from build123d import *

# Parameters (mm, degrees)
SKETCH_1_W                = 86
SKETCH_1_H                = 63
EXTRUDE_1_DEPTH           = 2
SKETCH_2_W                = 86
SKETCH_2_H                = 63
SKETCH_2_W_2              = 82
SKETCH_2_H_2              = 59
EXTRUDE_3_DEPTH           = 52.6
SKETCH_4_W                = 82
SKETCH_4_H                = 17.6
CUT_EXTRUDE_1_DEPTH       = 52.6
SKETCH_5_R                = 1.6
SKETCH_5_R_2              = 4.6
CUT_EXTRUDE_2_DEPTH       = 2
SKETCH_7_R                = 1.6
CUT_EXTRUDE_6_DEPTH       = 2
SKETCH_8_R                = 1.6
SKETCH_8_R_2              = 1.516132991
CUT_EXTRUDE_7_DEPTH       = 2
SKETCH_9_W                = 63
SKETCH_9_H                = 54.6
EXTRUDE_4_DEPTH           = 5
SKETCH_10_R               = 1.6
SKETCH_10_R_2             = 4.6
CUT_EXTRUDE_8_DEPTH       = 5
CUT_EXTRUDE_START         = -5
SKETCH_11_R               = 1.6
SKETCH_11_R_2             = 4.6
CUT_EXTRUDE_9_DEPTH       = 5
SKETCH_12_W               = 5
SKETCH_12_H               = 15.6
EXTRUDE_5_DEPTH           = 2
SKETCH_13_R               = 2.787491564
CUT_EXTRUDE_10_DEPTH      = 2
SKETCH_14_R               = 3
CUT_EXTRUDE_11_DEPTH      = 2
SKETCH_16_W               = 9
SKETCH_16_H               = 3.75891244
SKETCH_16_H_2             = 3.76
EXTRUDE_6_DEPTH           = 6
CUT_EXTRUDE_15_DEPTH      = 80.341453127
CUT_EXTRUDE_15_DEPTH_BACK = 80.341453127
SKETCH_17_R               = 1.6
SKETCH_18_W               = 9
SKETCH_18_H               = 6
SKETCH_18_R               = 1.6
EXTRUDE_7_DEPTH           = 3.76


with BuildPart() as part:
    # 草图1 → 凸台-拉伸1 (new body)
    with BuildSketch(Plane(origin=(0, 0, 0), x_dir=(1, 0, 0), z_dir=(0, 1, 0))):
        Rectangle(SKETCH_1_W, SKETCH_1_H)
    extrude(amount=EXTRUDE_1_DEPTH)

    # 草图2 → 凸台-拉伸3 (add)
    with BuildSketch(Plane(origin=(0, 2, 0), x_dir=(1, 0, 0), z_dir=(0, 1, 0))):
        Rectangle(SKETCH_2_W, SKETCH_2_H)
        Rectangle(SKETCH_2_W_2, SKETCH_2_H_2, mode=Mode.SUBTRACT)
    extrude(amount=EXTRUDE_3_DEPTH)

    # 草图4 → 切除-拉伸1 (cut)
    with BuildSketch(Plane.XY.offset(-29.5)):
        with Locations((0, 45.8)):
            Rectangle(SKETCH_4_W, SKETCH_4_H)
    extrude(amount=-CUT_EXTRUDE_1_DEPTH, mode=Mode.SUBTRACT)

    # 草图5 → 切除-拉伸2 (cut)
    with BuildSketch(Plane(origin=(43, 0, 0), x_dir=(0, 0, -1), z_dir=(1, 0, 0))):
        with Locations((-17.5, 16.95452537)):
            Circle(SKETCH_5_R)
        with Locations((17.5, 16.95452537)):
            Circle(SKETCH_5_R)
        with Locations((0, 8.95452537)):
            Circle(SKETCH_5_R_2)
    extrude(amount=-CUT_EXTRUDE_2_DEPTH, mode=Mode.SUBTRACT)

    # 草图7 → 切除-拉伸6 (cut)
    with BuildSketch(Plane(origin=(0, 2, 0), x_dir=(1, 0, 0), z_dir=(0, 1, 0))):
        with Locations(Location((-38.17, 6.16, 0), (0, 0, 270))):
            Circle(SKETCH_7_R)
        with Locations(Location((-38.17, -26.73, 0), (0, 0, 270))):
            Circle(SKETCH_7_R)
        with Locations(Location((36.38, -26.73, 0), (0, 0, 270))):
            Circle(SKETCH_7_R)
    extrude(amount=-CUT_EXTRUDE_6_DEPTH, mode=Mode.SUBTRACT)

    # 草图8 → 切除-拉伸7 (cut)
    with BuildSketch(Plane(origin=(0, 2, 0), x_dir=(1, 0, 0), z_dir=(0, 1, 0))):
        with Locations(Location((-39, 1.715, 0), (0, 0, 270))):
            Circle(SKETCH_8_R)
        with Locations(Location((21, -22.285, 0), (0, 0, 270))):
            Circle(SKETCH_8_R)
        with Locations(Location((-39, -22.285, 0), (0, 0, 270))):
            Circle(SKETCH_8_R_2)
        with Locations(Location((21, 1.715, 0), (0, 0, 270))):
            Circle(SKETCH_8_R)
    extrude(amount=-CUT_EXTRUDE_7_DEPTH, mode=Mode.SUBTRACT)

    # 草图9 → 凸台-拉伸4 (add)
    with BuildSketch(Plane(origin=(43, 0, 0), x_dir=(0, 0, -1), z_dir=(1, 0, 0))):
        with Locations((0, 27.3)):
            Rectangle(SKETCH_9_W, SKETCH_9_H)
    extrude(amount=EXTRUDE_4_DEPTH)

    # 草图10 → 切除-拉伸8 (cut)
    with BuildSketch(Plane(origin=(48, 0, 0), x_dir=(0, 0, -1), z_dir=(1, 0, 0))):
        with Locations((-17.5, 16.95452537)):
            Circle(SKETCH_10_R)
        with Locations((0, 8.95452537)):
            Circle(SKETCH_10_R_2)
        with Locations((17.5, 16.95452537)):
            Circle(SKETCH_10_R)
    extrude(amount=-CUT_EXTRUDE_8_DEPTH, mode=Mode.SUBTRACT)

    # 草图11 → 切除-拉伸9 (cut)
    with BuildSketch(Plane.ZY.offset(-41).offset(CUT_EXTRUDE_START)):
        Polygon((29.5, 52.6), (-31.5, 52.6), (-31.5, 37), (-29.5, 37), (-29.5, 2), (29.5, 2), align=None)
        with Locations(Location((-17.5, 16.95452537, 0), (0, 0, 180))):
            Circle(SKETCH_11_R, mode=Mode.SUBTRACT)
        with Locations(Location((0, 8.95452537, 0), (0, 0, 180))):
            Circle(SKETCH_11_R_2, mode=Mode.SUBTRACT)
        with Locations(Location((17.5, 16.95452537, 0), (0, 0, 180))):
            Circle(SKETCH_11_R, mode=Mode.SUBTRACT)
    extrude(amount=CUT_EXTRUDE_9_DEPTH, mode=Mode.SUBTRACT)

    # 草图12 → 凸台-拉伸5 (add)
    with BuildSketch(Plane(origin=(0, 0, -31.5), x_dir=(-1, 0, 0), z_dir=(0, 0, -1))):
        with Locations((-43.5, 44.8)):
            Rectangle(SKETCH_12_W, SKETCH_12_H)
    extrude(amount=-EXTRUDE_5_DEPTH)

    # 草图13 → 切除-拉伸10 (cut)
    with BuildSketch(Plane(origin=(48, 0, 0), x_dir=(0, 0, -1), z_dir=(1, 0, 0))):
        with Locations((24.963130904, 7.208902204)):
            Circle(SKETCH_13_R)
    extrude(amount=-CUT_EXTRUDE_10_DEPTH, mode=Mode.SUBTRACT)

    # 草图14 → 切除-拉伸11 (cut)
    with BuildSketch(Plane(origin=(0, 0, -31.5), x_dir=(-1, 0, 0), z_dir=(0, 0, -1))):
        with Locations((-28.059363277, 7.365425106)):
            Circle(SKETCH_14_R)
    extrude(amount=-CUT_EXTRUDE_11_DEPTH, mode=Mode.SUBTRACT)

    # 草图16 → 凸台-拉伸6 (add)
    with BuildSketch(Plane(origin=(0, 0, -31.5), x_dir=(-1, 0, 0), z_dir=(0, 0, -1))):
        with Locations((34.110668407, 1.87945622)):
            Rectangle(SKETCH_16_W, SKETCH_16_H)
        with Locations((-7.158197826, 1.88)):
            Rectangle(SKETCH_16_W, SKETCH_16_H_2)
    extrude(amount=EXTRUDE_6_DEPTH)

    # 草图17 → 切除-拉伸15 (cut, two sides: drawn at the far end of the back side and taken through both)
    with BuildSketch(Plane(origin=(0, 3.75891244, 0), x_dir=(1, 0, 0), z_dir=(0, 1, 0)).offset(-CUT_EXTRUDE_15_DEPTH_BACK)):
        with Locations(Location((-34.110668407, 34.625200871, 0), (0, 0, 180))):
            Circle(SKETCH_17_R)
        with Locations(Location((7.158197826, 34.625200871, 0), (0, 0, 180))):
            Circle(SKETCH_17_R)
    extrude(amount=CUT_EXTRUDE_15_DEPTH + CUT_EXTRUDE_15_DEPTH_BACK, mode=Mode.SUBTRACT)

    # 草图18 → 凸台-拉伸7 (add)
    # profile 1 of 2: a face of its own
    with BuildSketch(Plane.XZ):
        with Locations((7.158197826, 34.5)):
            Rectangle(SKETCH_18_W, SKETCH_18_H)
        with Locations(Location((7.158197826, 34.625200871, 0), (0, 0, 270))):
            Circle(SKETCH_18_R, mode=Mode.SUBTRACT)
    # profile 2 of 2: a face of its own
    with BuildSketch(Plane.XZ):
        with Locations((-34.110668407, 34.5)):
            Rectangle(SKETCH_18_W, SKETCH_18_H)
        with Locations(Location((-34.110668407, 34.625200871, 0), (0, 0, 270))):
            Circle(SKETCH_18_R, mode=Mode.SUBTRACT)
    extrude(amount=-EXTRUDE_7_DEPTH)


solid = part.part
Can you work these out from the model? Positions are in its coordinate system, mm. A direction names the side the tool comes from. Give positions to 0.01 mm unless a question says otherwise; leave off trailing zeros. Loops run counter-clockwise (first coordinate to the right, second up) from the corner with the lowest first, then second, coordinate; pieces in that order, holes last. Notation, with made-up numbers: (-18, -4.5) - (12, -4.5) arc R15 cw to (12, 15.5) - close; hole circle Ø2 at (22.25, 30). An arc over 180 degrees is marked (long way). Answer as a JSON object with one key per item and string values.
Q1. If we mould it in two halves opening along Z, with no side actions, what happens to faces 1 (the cylindrical face through (-40.48, 1.01, 21.96)), 2 (the cylindrical face through (-36.584, 1.014, -6.368)), 3 (the flat face through (41, 53, -8)), 4 (the flat face through (-34, 2, -37.5))? For each: pulls with the +Z half, pulls with the -Z half, needs draft (parallel to the pull), parting line crosses it, or undercut.
Geometry says:
{"face 1": "undercut", "face 2": "undercut", "face 3": "needs draft", "face 4": "pulls with the -Z half"}
Q2. Imagine slicing it at A-A on z = 17.5. Write out the boundary of the cut face in (x, y), plus the area to 3 significant figures.
Geometry says:
{"outline": "(-43, 0) - (48, 0) - (48, 15.35) - (46, 15.35) - (46, 2) - (-41, 2) - (-41, 54.6) - (-43, 54.6) - close; (41, 52.6) - (46, 52.6) - (46, 18.55) - (48, 18.55) - (48, 54.6) - (41, 54.6) - close", "area": "396 mm²"}
Q3. If I drill on L1, parallel to X at y = 10.5, z = -12; L2, parallel to Y at x = 46.9, z = -17.5; L3, parallel to Y at x = 42.5, z = -6.5, over which ranges is the centre line in solid material (lowest first)?
Geometry says:
{"L1": "-43 to -41, 46 to 48", "L2": "0 to 15.35, 18.55 to 54.6", "L3": "0 to 2, 52.6 to 54.6"}
Q4. Imagine slicing it at D-D on y = 38.5. Write out the boundary of the cut face in (x, z), plus the area to 3 significant figures.
Geometry says:
{"outline": "(-43, -31.5) - (-41, -31.5) - (-41, 29.5) - (46, 29.5) - (46, -29.5) - (41, -29.5) - (41, -31.5) - (48, -31.5) - (48, 31.5) - (-43, 31.5) - close", "area": "436 mm²"}
Q5. Which directions (+Z, -Z, +X, -X, +Y, -Y) give clear straight access to the entire face, cutting with the end or side of a thin tool? Please do faces 5 (the flat face through (-29.611, 2, -34)), 6 (the flat face through (44, 52.6, 0)), 7 (the flat face through (2.658, 2, 34)), 8 (the flat face through (-1, 37, -30)), 9 (the cylindrical face through (47.014, 18.036, 18.679)).
Geometry says:
{"face 5": "-Z, +Y, -Y", "face 6": "none", "face 7": "+Z, +Y, -Y", "face 8": "-Z, +Y", "face 9": "+X"}
Q6. Will these pins go through, and if not, where does the flat tip stop? P1, Ø5, axis at x = 37, y = 11.5, coming from the -Z side; P2, Ø3, axis at y = 2.5, z = 34.5, coming from the +X side; P3, Ø2.5, axis at x = -39, z = 22.285, coming from the -Y side; P4, Ø4, axis at y = 2, z = 34, coming from the -X side.
Geometry says:
{"P1": "z = -31.5", "P2": "x = 11.66", "P3": "through", "P4": "x = -38.61"}
Q7. Imagine slicing it at B-B on x = 21. Write out the boundary of the cut face in (y, z) (3 decimals).
Geometry says:
{"outline": "(0, -31.5) - (37, -31.5) - (37, -29.5) - (2, -29.5) - (2, -3.315) - (0, -3.315) - close; (0, -0.115) - (2, -0.115) - (2, 20.685) - (0, 20.685) - close; (0, 23.885) - (2, 23.885) - (2, 29.5) - (54.6, 29.5) - (54.6, 31.5) - (0, 31.5) - close"}
Q8. Imagine slicing it at C-C on z = 26.73. Write out the boundary of the cut face in (x, y), plus the area to 3 significant figures.
Geometry says:
{"outline": "(-43, 0) - (-39.77, 0) - (-39.77, 2) - (-41, 2) - (-41, 54.6) - (-43, 54.6) - close; (-36.57, 0) - (34.78, 0) - (34.78, 2) - (-36.57, 2) - close; (37.98, 0) - (48, 0) - (48, 54.6) - (41, 54.6) - (41, 52.6) - (46, 52.6) - (46, 2) - (37.98, 2) - close", "area": "390 mm²"}
